Part print with two shaded views. Sizes in mm from the minimum x, y, z corner. Round coordinates to 2 decimals unless told otherwise and drop trailing zeros. Order: outer loops, then holes, each group sorted by start corner. A loop starts at its lowest first (then second) coordinate and runs counter-clockwise, first axis right, second up. Notation, with made-up numbers: (15, 84) - (19, 84) arc R20 cw to (19, 117) - close; hole circle Ø8 at (7, -25.5). An arc over 180 degrees is marked (long way). Write item = value, one per line.
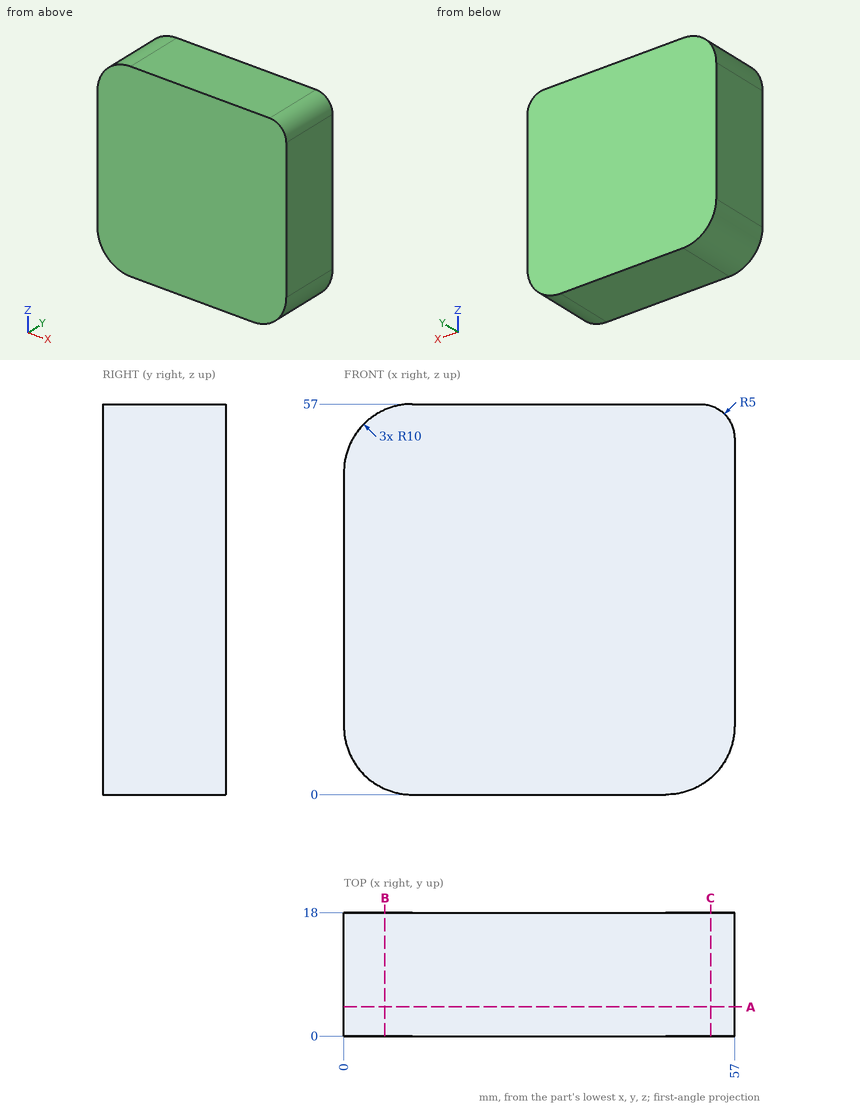
1) Cut at B-B (x = 6). Write the cut outline in (y, z).
Conclusion:
outline = (0, 0.83) - (18, 0.83) - (18, 56.17) - (0, 56.17) - close
2) Cut at A-A (y = 4.25). Write the cut outline in (x, z).
Conclusion:
outline = (0, 10) arc R10 ccw to (10, 0) - (47, 0) arc R10 ccw to (57, 10) - (57, 52) arc R5 ccw to (52, 57) - (10, 57) arc R10 ccw to (0, 47) - close
3) Flat gauge pin, fed straight in: pin 1 Ø4 at (x, z) = (16, 50.5) entering from -Y. Where does the tip first touch, or does it go through?
Conclusion:
pin_1 = 0
4) Cut at C-C (x = 53.5). Write the cut outline in (y, z), and give its area (3 significant figures).
Conclusion:
outline = (0, 2.4) - (18, 2.4) - (18, 56.77) - (0, 56.77) - close
area = 979 mm^2
5) Wall check: line 1 along Z through (x, y) = (49, 3.75); line 2 along Z through (x, y) = (6, 1.25); line 3 along X through (y, z) = (16.75, 51). Give the ranges that are in metal, low to high.
Conclusion:
line_1 = 0.2 to 57
line_2 = 0.83 to 56.17
line_3 = 0.83 to 57
